The listing builds one solid part. Answer for the finished solid, in the listing's coordinates (mm). Face numbers are marked on the shaded views. A direction names the side the tool comes from. Coordinates: 2 decimals unless noted, no trailing zeros. Loops run counter-clockwise (first coordinate to the right, second up) from the corner with the lowest first, then second, coordinate; pieces in that order, holes last. Notation, with made-up numbers: M 31,-14.75 L 41,-14.75 A15 ccw 41,1.25 Z; hole C -29,52.25 d5. An arc over 180 degrees is marked long. Return JSON: item names as keys, results as strings. Group by question number.
1. Section C-C (y = 0.5) is taken. Write down the section's boundary in (x, z).
2. Section B-B (z = -8.95) is taken. Write down the section's boundary in (x, y), then the cut area to 3 significant figures.
3. Which of the six approach directions +Z, -Z, +X, -X, +Y, -Y give full straight-line access (tool end or side, diameter ignored) to the marked faces 1 and 2?
4. Section D-D (x = 0) is taken. Write down the section's boundary in (y, z), then the cut area to 3 significant figures.
5. Straight lines are drawn through the part: L1, parallel to Z at x = -9.95, y = 1.15; L2, parallel to X at y = 0.5, z = 8.95; L3, parallel to Y at x = -10, z = 2.5. For each, find the intervals that lie inside material, in ascending order. Write a range as from..to.
6. Section A-A (x = -9.95) is taken. Write down the section's boundary in (y, z).
7. Given P1, Ø3, axis at x = -9.95, z = -8.95, coming from the +Y side; P2, Ø12, axis at x = 7.5, z = 8.5, coming from the +Y side; P3, Ø1.5, axis at x = 4, y = 4.5, coming from the +Z side, each flat-ended and moving along its own axis, determine where each tip first touches the part or whether it passes through.
```python
from build123d import *

# Parameters (mm, degrees)
SKETCH1_W           = 25.4
SKETCH1_H           = 23.4
BOSS_EXTRUDE1_DEPTH = 1.64
SKETCH2_R           = 1.75
CUT_EXTRUDE1_DEPTH  = 2.64
SKETCH3_R           = 4.85
BOSS_EXTRUDE2_DEPTH = 4.53
FILLET1_R           = 0.5


with BuildPart() as part:
    # Sketch1 → Boss-Extrude1 (new body)
    with BuildSketch(Plane(origin=(0, 0, 0), x_dir=(1, 0, 0), z_dir=(0, 1, 0))):
        Rectangle(SKETCH1_W, SKETCH1_H)
    extrude(amount=BOSS_EXTRUDE1_DEPTH)

    # Sketch2 → Cut-Extrude1 (cut, through all)
    with BuildSketch(Plane(origin=(0, 1.64, 0), x_dir=(1, 0, 0), z_dir=(0, 1, 0))):
        with Locations((-9.95, -8.95)):
            Circle(SKETCH2_R)
        with Locations((9.95, -8.95)):
            Circle(SKETCH2_R)
        with Locations((9.95, 8.95)):
            Circle(SKETCH2_R)
        with Locations((-9.95, 8.95)):
            Circle(SKETCH2_R)
    extrude(amount=-CUT_EXTRUDE1_DEPTH, mode=Mode.SUBTRACT)

    # Sketch3 → Boss-Extrude2 (add)
    with BuildSketch(Plane(origin=(0, 1.64, 0), x_dir=(1, 0, 0), z_dir=(0, 1, 0))):
        Circle(SKETCH3_R)
    extrude(amount=BOSS_EXTRUDE2_DEPTH)

    # Fillet1
    fillet1_edges = [part.edges().sort_by_distance(p)[0] for p in [
        (-4.85, 6.17, 0),
    ]]
    fillet(fillet1_edges, radius=FILLET1_R)


solid = part.part
```
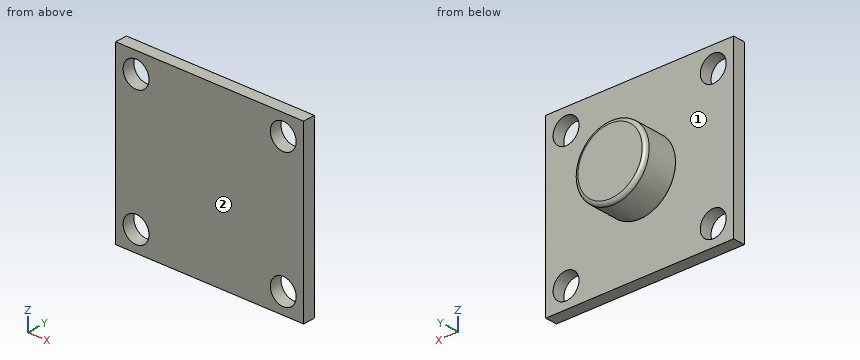
Worked out:
{
 "1": {"outline": "M -12.7,-11.7 L 12.7,-11.7 L 12.7,11.7 L -12.7,11.7 Z; hole C -9.95,-8.95 d3.5; hole C -9.95,8.95 d3.5; hole C 9.95,-8.95 d3.5; hole C 9.95,8.95 d3.5"},
 "2": {"outline": "M -12.7,0 L -11.7,0 L -11.7,1.64 L -12.7,1.64 Z; M -8.2,0 L 8.2,0 L 8.2,1.64 L -8.2,1.64 Z; M 11.7,0 L 12.7,0 L 12.7,1.64 L 11.7,1.64 Z", "area": "30.2 mm^2"},
 "3": {"face 1": "+Y", "face 2": "+Z, -Z, +X, -X, -Y"},
 "4": {"outline": "M 0,-11.7 L 1.64,-11.7 L 1.64,-4.85 L 5.67,-4.85 A0.5 ccw 6.17,-4.35 L 6.17,4.35 A0.5 ccw 5.67,4.85 L 1.64,4.85 L 1.64,11.7 L 0,11.7 Z", "area": "82.2 mm^2"},
 "5": {"L1": "-11.7..-10.7, -7.2..7.2, 10.7..11.7", "L2": "-12.7..-11.7, -8.2..8.2, 11.7..12.7", "L3": "0..1.64"},
 "6": {"outline": "M 0,-11.7 L 1.64,-11.7 L 1.64,-10.7 L 0,-10.7 Z; M 0,-7.2 L 1.64,-7.2 L 1.64,7.2 L 0,7.2 Z; M 0,10.7 L 1.64,10.7 L 1.64,11.7 L 0,11.7 Z"},
 "7": {"P1": "through", "P2": "y = 1.64", "P3": "z = 3.6"}
}
